Build history of the part. All positions in model axes, mm. A direction names the side the tool comes from. Round coordinates to 2 decimals unless told otherwise and drop trailing zeros. Loops run counter-clockwise (first coordinate to the right, second up) from the corner with the lowest first, then second, coordinate; pieces in that order, holes last. Notation, with made-up numbers: (79, 20) - (131, 20) arc R29 ccw to (131, 50) - close; hole circle Ø1 at (23.5, 80.25). An arc over 180 degrees is marked (long way). Use one line per item in the form item = value. Start each with the question number.
Q1. Drill centre lines: line 1 (X direction, y = 1.75, z = 37.25); line 2 (Y direction, x = 1.25, z = 39); line 3 (Y direction, x = 2.75, z = 39). Where is each one in solid material? Low to high.
Q2. Saw through at B-B (x = 0.25). Give the cut face in (y, z), then the cut area to 3 significant figures.
Q3. Saw through at C-C (z = 30.75). Give the cut face in (x, y), then the cut area to 3 significant figures.
Q4. 3-axis set-ups, long thin cutter, end or side, ignore diameter. For faces 1 (the face through (4, 12.5, 31)), 2 (the face through (2, 0, 31)): which of +Z, -Z, +X, -X, +Y, -Y reach the whole face in a straight line?
Q5. Saw through at A-A (y = 1.5). Give the cut face in (x, z).
Q6. Saw through at D-D (x = 3.25). Give the cut face in (y, z), then the cut area to 3 significant figures.
Q7. Mould opens along X. For faces 3 (the face through (5.2, 6, 40)), 4 (the face through (5.5, 6, 31)), 5 (the face through (0, 6, 31)) say: released by +X, released by -X, zero draft, split by the parting line, or undercut.
```python
from build123d import *

# Parameters (mm, degrees)
EXTRUDE_1_DEPTH     = 40
SKETCH_2_R          = 22.5
CUT_EXTRUDE_1_DEPTH = 40


with BuildPart() as part:
    # ｽｹｯﾁ1 → ﾎﾞｽ - 押し出し1 (new body)
    with BuildSketch(Plane.XY):
        Polygon((0, 0), (5, 0), (5, 12), (3.5, 12), (3.5, 12.5), (5.5, 12.5), (5.5, 12), (5.5, -0.5), (-0.5, -0.5), (-0.5, 12), (-0.5, 12.5), (1.5, 12.5), (1.5, 12), (0, 12), align=None)
    extrude(amount=EXTRUDE_1_DEPTH)

    # ｽｹｯﾁ2 → ｶｯﾄ - 押し出し1 (cut)
    with BuildSketch(Plane.XZ.offset(0.5)):
        with Locations((2.5, 0)):
            Circle(SKETCH_2_R)
    extrude(amount=-CUT_EXTRUDE_1_DEPTH, mode=Mode.SUBTRACT)


solid = part.part
```
Report:
q1.line_1 = -0.5 to 0, 5 to 5.5
q1.line_2 = -0.5 to 0, 12 to 12.5
q1.line_3 = -0.5 to 0
q2.outline = (-0.5, 22.39) - (0, 22.39) - (0, 40) - (-0.5, 40) - close; (12, 22.39) - (12.5, 22.39) - (12.5, 40) - (12, 40) - close
q2.area = 17.6 mm²
q3.outline = (-0.5, -0.5) - (5.5, -0.5) - (5.5, 12.5) - (3.5, 12.5) - (3.5, 12) - (5, 12) - (5, 0) - (0, 0) - (0, 12) - (1.5, 12) - (1.5, 12.5) - (-0.5, 12.5) - close
q3.area = 17.0 mm²
q4.face_1 = +Z, -Z, +X, -X, +Y
q4.face_2 = +Z, -Z
q5.outline = (-0.5, 22.3) arc R22.5 cw to (0, 22.36) - (0, 40) - (-0.5, 40) - close; (5, 22.36) arc R22.5 cw to (5.5, 22.3) - (5.5, 40) - (5, 40) - close
q6.outline = (-0.5, 22.49) - (0, 22.49) - (0, 40) - (-0.5, 40) - close
q6.area = 8.76 mm²
q7.face_3 = zero draft
q7.face_4 = released by +X
q7.face_5 = undercut
